Input: part model. Units: mm. Frame: model coordinates. A direction names the side the tool comes from. Round coordinates to 2 decimals unless told otherwise and drop trailing zeros. Order: outer loops, then holes, each group sorted by start corner. A loop starts at its lowest first (then second) coordinate and runs counter-clockwise, first axis right, second up. Notation, with made-up numbers: (19.25, 86.25) -> (42.25, 86.25) arc R24 ccw to (42.25, 109.25) -> close; hole circle Ø10 at (61.5, 33.5). An arc over 180 degrees is marked (long way). Answer as CSV lines item,"result". Start each with the question number.
1) Mould query, pull axis X, two halves, no side actions, for faces 1 (the face through (24, -5, 207)), 2 (the face through (-7.535, -23.05, 206.57)), 3 (the face through (-11.18, -19.5, 206.57)), 4 (the face through (12.46, -22.2, 206.22)). Classes: +X half, -X half, draft (parallel to the pull), parting line (faces both ways), or undercut.
2) Section query A-A, the plane x = -12. Output: boundary loops of the cut face in (y, z), and give its area (3 significant figures).
3) First-contact query: P1, Ø1.6, axis at x = -6.5, z = 206, coming from the -Y side. Flat tip, straight axial feed; report the tip coordinate or a pass-through.
4) Section query C-C, the plane y = -14. State how many separate pieces and enclosed holes the cut face has, and give its area (3 significant figures).
5) Line query: L1, parallel to X at y = -8, z = 206.6; L2, parallel to Y at x = -16, z = 206.85; L3, parallel to X at y = 3, z = 206.25. Output: solid intervals per line, ascending.
6) Access query for faces 5 (the face through (-25.455, 0.304, 206.216)), 6 (the face through (-9.763, -17.455, 206.57)). Directions: +Z, -Z, +X, -X, +Y, -Y. A direction counts if a zero-diameter tool reaches every point of the face in a straight line with its end or side. Return the directions, or none.
7) Section query B-B, the plane z = 205.65. Output: boundary loops of the cut face in (x, y), and give its area (3 significant figures).
```python
from build123d import *

# Parameters (mm, degrees)
CUT_EXTRUDE1_DEPTH = 5
CIRPATTERN1_COUNT  = 3
CUT_EXTRUDE2_DEPTH = 3.180622175


with BuildPart() as part:
    # Sketch1 → Revolve1 (revolve)
    with BuildSketch(Plane(origin=(0, 0, 0), x_dir=(1, 0, 0), z_dir=(0, 1, 0)), mode=Mode.PRIVATE) as revolve1_sk:
        Polygon((0, -208.182219687), (25.746837518, -208.182219687), (25.276959566, -205.001597513), (0, -205.001597513), align=None)
    revolve(revolve1_sk.sketch.rotate(Axis((0, 0, 0), (0, 0, 1)), 180), axis=Axis((0, 0, 0), (0, 0, 1)))

    # Sketch2 → Cut-Extrude1 (cut, symmetric)
    with BuildSketch(Plane(origin=(0, 0, 0), x_dir=(1, 0, 0), z_dir=(0, 1, 0))):
        Polygon((22.094125947, -203.98439075), (22.850570101, -209.104790721), (26.737620159, -209.104790721), (25.746837518, -203.98439075), align=None)
    cut_extrude1 = extrude(amount=CUT_EXTRUDE1_DEPTH, both=True, mode=Mode.SUBTRACT)

    # CirPattern1: Cut-Extrude1 ×3 about axis
    cirpattern1_axis = Axis((0, 0, 0), (0, 0, 1))
    for i in range(1, CIRPATTERN1_COUNT):
        add(cut_extrude1.rotate(cirpattern1_axis, i * 360 / CIRPATTERN1_COUNT), mode=Mode.SUBTRACT)

    # Sketch3 → Cut-Extrude2 (cut)
    with BuildSketch(Plane(origin=(0, 0, 205.001597513), x_dir=(-1, 0, 0), z_dir=(0, 0, -1))):
        with BuildLine():
            Line((-11.270873443, -16.521725449), (-2.299038106, -0.982050808))
            ThreePointArc((-2.299038106, -0.982050808), (-2.5, 0), (-2.299038106, 0.982050808))
            Line((-2.299038106, 0.982050808), (-11.270873443, 16.521725449))
            ThreePointArc((-11.270873443, 16.521725449), (-20, 0), (-11.270873443, -16.521725449))
        make_face()
        with BuildLine():
            ThreePointArc((19.943670675, 1.5), (10, 17.320508076), (-8.672797232, 18.021725449))
            Line((-8.672797232, 18.021725449), (0.299038106, 2.482050808))
            ThreePointArc((0.299038106, 2.482050808), (1.25, 2.165063509), (2, 1.5))
            Line((2, 1.5), (19.943670675, 1.5))
        make_face()
        with BuildLine():
            Line((0.299038106, -2.482050808), (-8.672797232, -18.021725449))
            ThreePointArc((-8.672797232, -18.021725449), (10, -17.320508076), (19.943670675, -1.5))
            Line((19.943670675, -1.5), (2, -1.5))
            ThreePointArc((2, -1.5), (1.25, -2.165063509), (0.299038106, -2.482050808))
        make_face()
    extrude(amount=-CUT_EXTRUDE2_DEPTH, mode=Mode.SUBTRACT)


solid = part.part
```
Findings:
1,face 1,"draft"
1,face 2,"-X half"
1,face 3,"undercut"
1,face 4,"parting line"
2,outline,"(-19.3, 208.18) -> (-18.76, 205) -> (-16, 205) -> (-16, 208.18) -> close; (-1.5, 205) -> (1.5, 205) -> (1.5, 208.18) -> (-1.5, 208.18) -> close; (16, 205) -> (18.76, 205) -> (19.3, 208.18) -> (16, 208.18) -> close"
2,area,"28.8 mm^2"
3,P1,"stops at y = -24.81"
4,separate pieces,"3"
4,enclosed holes,"0"
4,area,"55.8 mm^2"
5,L1,"x = -24.23 to -18.33, 2.89 to 6.35, 18.33 to 24.23"
5,L2,"y = -17.71 to -12, -1.5 to 1.5, 12 to 17.71"
5,L3,"x = -25.28 to -19.77, 0 to 3.46, 19.77 to 22.43"
6,face 5,"-Z, -X"
6,face 6,"+Z, -Z"
7,outline,"(-16.77, -19.04) -> (-15.5, -16.85) -> (-6.84, -21.85) -> (-8.11, -24.04) arc R25.37 ccw to (24.88, -5) -> (22.34, -5) -> (22.34, 5) -> (24.88, 5) arc R25.37 ccw to (-8.11, 24.04) -> (-6.84, 21.85) -> (-15.5, 16.85) -> (-16.77, 19.04) arc R25.37 ccw to start; hole (-19.94, -1.5) arc R20 ccw to (8.67, -18.02) -> (-0.3, -2.48) arc R2.5 cw to (-2, -1.5) -> close; hole (-19.94, 1.5) -> (-2, 1.5) arc R2.5 cw to (-0.3, 2.48) -> (8.67, 18.02) arc R20 ccw to start; hole (2.3, -0.98) -> (11.27, -16.52) arc R20 ccw to (11.27, 16.52) -> (2.3, 0.98) arc R2.5 cw to start"
7,area,"858 mm^2"
